```python
from build123d import *

# Parameters (mm, degrees)
BOSS_EXTRUDE1_DEPTH                     = 12
CBORE_FOR_M5_HEX_HEAD_BOLT1_D           = 8
CBORE_FOR_M5_HEX_HEAD_BOLT1_CBORE_D     = 10
CBORE_FOR_M5_HEX_HEAD_BOLT1_CBORE_DEPTH = 3.58
SKETCH4_R                               = 20
BOSS_EXTRUDE2_DEPTH                     = 53
BOSS_EXTRUDE3_DEPTH                     = 20
CBORE_FOR_M5_HEX_HEAD_BOLT5_D           = 10
CBORE_FOR_M5_HEX_HEAD_BOLT5_DEPTH       = 25
CBORE_FOR_M5_HEX_HEAD_BOLT5_CBORE_D     = 14
CBORE_FOR_M5_HEX_HEAD_BOLT5_CBORE_DEPTH = 18
CBORE_FOR_M5_HEX_HEAD_BOLT5_TIP         = 3.004303095
SKETCH11_W                              = 46
SKETCH11_H                              = 10
CUT_EXTRUDE1_DEPTH                      = 105.16333328


with BuildPart() as part:
    # Sketch2 → Boss-Extrude1 (new body)
    with BuildSketch(Plane(origin=(0, 0, 0), x_dir=(1, 0, 0), z_dir=(0, 1, 0))):
        with BuildLine():
            Line((-30, -22.5), (30, -22.5))
            ThreePointArc((30, -22.5), (37.071067812, -19.571067812), (40, -12.5))
            Line((40, -12.5), (40, 12.5))
            ThreePointArc((40, 12.5), (37.071067812, 19.571067812), (30, 22.5))
            Line((30, 22.5), (-30, 22.5))
            ThreePointArc((-30, 22.5), (-37.071067812, 19.571067812), (-40, 12.5))
            Line((-40, 12.5), (-40, -12.5))
            ThreePointArc((-40, -12.5), (-37.071067812, -19.571067812), (-30, -22.5))
        make_face()
    extrude(amount=BOSS_EXTRUDE1_DEPTH)

    # CBORE for M5 Hex Head Bolt1 (through all)
    with Locations(Plane(origin=(-30, 12, 12.5), x_dir=(0, 0, 1), z_dir=(0, 1, 0))):
        with Locations((0, 0), (-25, 0), (-25, 60), (0, 60)):
            CounterBoreHole(CBORE_FOR_M5_HEX_HEAD_BOLT1_D / 2, CBORE_FOR_M5_HEX_HEAD_BOLT1_CBORE_D / 2, CBORE_FOR_M5_HEX_HEAD_BOLT1_CBORE_DEPTH)

    # Sketch4 → Boss-Extrude2 (add)
    with BuildSketch(Plane(origin=(0, 12, 0), x_dir=(1, 0, 0), z_dir=(0, 1, 0))):
        with Locations(Location((0, 0, 0), (0, 0, 90))):
            Circle(SKETCH4_R)
    extrude(amount=BOSS_EXTRUDE2_DEPTH)

    # Sketch5 → Boss-Extrude3 (add)
    with BuildSketch(Plane(origin=(0, 65, 0), x_dir=(1, 0, 0), z_dir=(0, 1, 0))):
        Polygon((0, -14.142135624), (14.142135624, 0), (0, 14.142135624), (-14.142135624, 0), align=None)
    extrude(amount=BOSS_EXTRUDE3_DEPTH)

    # CBORE for M5 Hex Head Bolt5
    with Locations(Plane.ZX.offset(85)):
        with Locations((0, 0)):
            CounterBoreHole(CBORE_FOR_M5_HEX_HEAD_BOLT5_D / 2, CBORE_FOR_M5_HEX_HEAD_BOLT5_CBORE_D / 2, CBORE_FOR_M5_HEX_HEAD_BOLT5_CBORE_DEPTH, depth=CBORE_FOR_M5_HEX_HEAD_BOLT5_DEPTH)
            with Locations((0, 0, -(CBORE_FOR_M5_HEX_HEAD_BOLT5_DEPTH + CBORE_FOR_M5_HEX_HEAD_BOLT5_TIP / 2))):  # 118° drill point
                Cone(0, CBORE_FOR_M5_HEX_HEAD_BOLT5_D / 2, CBORE_FOR_M5_HEX_HEAD_BOLT5_TIP, mode=Mode.SUBTRACT)

    # Sketch10 → Cut-Revolve1 (revolve, cut)
    with BuildSketch(Plane.XY):
        with BuildLine():
            Line((0, 0), (0, 54))
            ThreePointArc((0, 54), (-9.899494937, 49.899494937), (-14, 40))
            Line((-14, 40), (-14, 0))
            Line((-14, 0), (0, 0))
        make_face()
    revolve(axis=Axis((0, 0, 0), (0, 1, 0)), mode=Mode.SUBTRACT)

    # Sketch11 → Cut-Extrude1 (cut, through all)
    with BuildSketch(Plane.XY.offset(22.5)):
        Rectangle(SKETCH11_W, SKETCH11_H)
    extrude(amount=-CUT_EXTRUDE1_DEPTH, mode=Mode.SUBTRACT)


solid = part.part
```
CAD build for the part. Positions are in the model's coordinates, mm. A direction names the side the tool comes from. Give positions to 0.01 mm unless a question says otherwise; leave off trailing zeros. Order: outer loops, then holes, each group sorted by start corner. A loop starts at its lowest first (then second) coordinate and runs counter-clockwise, first axis right, second up. Notation, with made-up numbers: M 52.25,23.5 L 102.25,23.5 A20 cw 102.25,41.5 Z; hole C 47.5,-21 d8. An arc over 180 degrees is marked long. Put each result on its own line as item: value. Start each with the question number.
(1) Flat gauge pins, fed straight in: pin 1 Ø5 at (y, z) = (24.5, -5) entering from -X; pin 2 Ø6 at (x, z) = (15.5, 5.5) entering from +Y; pin 3 Ø3 at (x, z) = (28, 10.5) entering from +Y. Where does each tip first touch, or does it go through?
(2) Mould opens along Z. For faces 4 (the cylindrical face through (33.966, 4.151, -11.979)), 5 (the flat face through (-6.97, 74.86, -7.17)), 6 (the cylindrical face through (33.966, 4.151, 13.021)), 7 (the flat face through (-40, 6, 0)) say: +Z half, -Z half, draft (parallel to the pull), parting line (faces both ways), or undercut.
(3) Which spindle directions (+Z, -Z, +X, -X, +Y, -Y) get a long thin tool onto all of the face, cutting with end or side? Do faces 1 (the flat face through (34, 8.42, 14)), 2 (the flat face through (-23, 2, 0)), 3 (the cylindrical face through (-12.932, 22.255, -5.362)). Say none if no direction does.
(4) Saw through at A-A, the plane y = 75.5. Write the cut outline in (x, z).
(5) Saw through at B-B, the plane y = 48. Write the cut outline in (x, z), then the cut area to 3 significant figures.
(6) Drill centre lines: line 1 along X through (y, z) = (3.25, 12.5); line 2 along X through (y, z) = (9.35, 12.5); line 3 along X through (y, z) = (19.5, 0). Where is each one in solid material? Low to high.
Check result:
1. pin 1: stops at x = -19.84
1. pin 2: stops at y = 65
1. pin 3: stops at y = 8.42
2. face 4: undercut
2. face 5: -Z half
2. face 6: undercut
2. face 7: draft
3. face 1: +Y
3. face 2: +Z, -Z, -Y
3. face 3: -Y
4. outline: M -14.14,0 L 0,-14.14 L 14.14,0 L 0,14.14 Z; hole C 0,0 d14
5. outline: C 0,0 d40; hole C 0,0 d22.98
5. area: 842 mm2
6. line 1: x = -40 to -34, -26 to -23, 23 to 26, 34 to 40
6. line 2: x = -40 to -35, -25 to -6.3, 6.3 to 25, 35 to 40
6. line 3: x = -20 to -14, 14 to 20
